Geometry: final body of the model. Coordinates: model frame, mm. A direction names the side the tool comes from. Coordinates: 2 decimals unless noted, no trailing zeros. Loops run counter-clockwise (first coordinate to the right, second up) from the corner with the lowest first, then second, coordinate; pieces in that order, holes last. Notation, with made-up numbers: (13.25, -8) - (34.25, -8) arc R16 ccw to (34.25, -1) - close; hole circle Ø11 at (-27.75, -26). An arc over 180 degrees is marked (long way). Write each question's results on one line, items separated by ' | '. Start each with the question number.
Autodesk Inventor part; units mm, degrees
ref_plane "YZ Plane" through (0, 0, 0) normal (1, 0, 0) x (0, 1, 0)
ref_plane "XZ Plane" through (0, 0, 0) normal (0, 1, 0) x (-1, 0, 0)
ref_plane "XY Plane" through (0, 0, 0) normal (0, 0, 1) x (1, 0, 0)
sketch "Sketch1" plane through (0, 0, 0) normal (0, 0, 1) x (1, 0, 0)
  line L0 (0, 0) -> (35, 0)
  line L1 (35, 0) -> (35, 35)
  line L2 (35, 35) -> (0, 35)
  line L3 (0, 35) -> (0, 0)
  line L4 (4.5, 30.5) -> (30.5, 30.5) construction
  line L5 (30.5, 30.5) -> (30.5, 4.5) construction
  line L6 (30.5, 4.5) -> (4.5, 4.5) construction
  line L7 (4.5, 4.5) -> (4.5, 30.5) construction
  circle A0 centre (4.5, 30.5) radius 1.5
  circle A1 centre (30.5, 30.5) radius 1.5
  circle A2 centre (30.5, 4.5) radius 1.5
  circle A3 centre (4.5, 4.5) radius 1.5
  circle A4 centre (17.5, 17.5) radius 2.5
  point P0 (17.5, 35)
  point P1 (35, 17.5)
  dimension "d0" = 35
  dimension "d1" = 35
  dimension "d2" = 26
  dimension "d3" = 3
  dimension "d4" = 3
  dimension "d5" = 3
  dimension "d6" = 3
  dimension "d9" = 5
extrude "Extrusion1" add sketch "Sketch1" along normal blind 28
chamfer "Chamfer1" distance 3 angle 45 4 edges at (35, 35, 14) (35, 0, 14) (0, 0, 14) (0, 35, 14)
sketch "Sketch2" plane through (0, 0, 28) normal (0, 0, 1) x (1, 0, 0)
  circle A0 centre (17.5, 17.5) radius 2.5 construction
  circle A1 centre (17.5, 17.5) radius 10
  point P0 (0, 0)
  dimension "d13" = 20
sketch "Sketch3" plane through (0, 0, 28) normal (0, 0, 1) x (1, 0, 0)
  circle A0 centre (17.5, 17.5) radius 2.5
  point P0 (0, 0)
extrude "Extrusion2" add sketch "Sketch3" along normal blind 25
extrude "Extrusion3" add sketch "Sketch2" along normal blind 2
properties part number "NEMA17"
1) Section query C-C on z = 20. Output: boundary loops of the cut face in (x, y), and give its area (3 significant figures).
2) Pin query (flat end, axial travel): pin 1 Ø3.5 at (x, y) = (4.5, 4.5) entering from -Z; pin 2 Ø1.5 at (x, y) = (14, 17) entering from +Z; pin 3 Ø5 at (x, y) = (4.5, 30.5) entering from +Z. Return the tip coordinate at first contact, or that it passes through.
3) Pull-direction query (Y, two-part tool) for faces 1 (the flat face through (35, 17, 14)), 2 (the flat face through (2, 34, 14)), 3 (the cylindrical face through (29, 4.43, 13.8)), 4 (the flat face through (33, 1, 14)); classes: released by +Y, released by -Y, zero draft, split by the parting line, or undercut.
4) Access query for faces 5 (the flat face through (0, 18, 14)), 6 (the flat face through (9, 10, 28)), 7 (the cylindrical face through (15, 17.4, 13.8)). Directions: +Z, -Z, +X, -X, +Y, -Y. A direction counts if a zero-diameter tool reaches every point of the face in a straight line with its end or side. Return the directions, or none.
5) Material intervals for line 1 (Y direction, x = 4.5, z = 10.25); line 2 (X direction, y = 30, z = 7), sorted ascending. Write a range as [from, to].
6) Section query A-A on y = 30.5. Output: boundary loops of the cut face in (x, z).
7) Section query D-D on x = 17.5. Output: boundary loops of the cut face in (y, z).
Returned:
1) outline: (0, 3) - (3, 0) - (32, 0) - (35, 3) - (35, 32) - (32, 35) - (3, 35) - (0, 32) - close; hole circle Ø3 at (4.5, 4.5); hole circle Ø3 at (4.5, 30.5); hole circle Ø5 at (17.5, 17.5); hole circle Ø3 at (30.5, 4.5); hole circle Ø3 at (30.5, 30.5) | area: 1,160 mm²
2) pin 1: stops at z = 0 | pin 2: stops at z = 30 | pin 3: stops at z = 28
3) face 1: zero draft | face 2: released by +Y | face 3: undercut | face 4: released by -Y
4) face 5: +Z, -Z, -X, +Y, -Y | face 6: +Z | face 7: -Z
5) line 1: y = [0, 3], [6, 29], [32, 35] | line 2: x = [0, 3.09], [5.91, 29.09], [31.91, 35]
6) outline: (0, 0) - (3, 0) - (3, 28) - (0, 28) - close; (6, 0) - (29, 0) - (29, 28) - (6, 28) - close; (32, 0) - (35, 0) - (35, 28) - (32, 28) - close
7) outline: (0, 0) - (15, 0) - (15, 28) - (20, 28) - (20, 0) - (35, 0) - (35, 28) - (27.5, 28) - (27.5, 30) - (20, 30) - (20, 53) - (15, 53) - (15, 30) - (7.5, 30) - (7.5, 28) - (0, 28) - close
